from build123d import *

# Parameters (mm, degrees)
BOSS_EXTRUDE3_DEPTH      = 62.5
BOSS_EXTRUDE3_DEPTH_BACK = 62.5
SKETCH4_R                = 1.8
CUT_EXTRUDE1_DEPTH       = 62.5
SKETCH5_R                = 1.8
CUT_EXTRUDE2_DEPTH       = 62.5
SKETCH7_W                = 21.5
SKETCH7_H                = 18
CUT_EXTRUDE5_DEPTH       = 62.5
SKETCH10_W               = 21.5
SKETCH10_H               = 18
CUT_EXTRUDE7_DEPTH       = 62.5
SKETCH13_W               = 21.5
SKETCH13_H               = 28.5
CUT_EXTRUDE9_DEPTH       = 62.5
SKETCH18_W               = 21.5
SKETCH18_H               = 28.5
CUT_EXTRUDE10_DEPTH      = 62.5
SKETCH20_R               = 1.7
CUT_EXTRUDE11_DEPTH      = 62.5
SKETCH21_R               = 1.7
CUT_EXTRUDE12_DEPTH      = 62.5


with BuildPart() as part:
    # Sketch1 → Boss-Extrude3 (new, two sides: drawn at the far end of the back side and taken through both)
    with BuildSketch(Plane.XY.offset(-BOSS_EXTRUDE3_DEPTH_BACK)):
        Polygon((0, 0), (0, 40), (3.5, 40), (3.5, 3.5), (25, 3.5), (25, 0), align=None)
    extrude(amount=BOSS_EXTRUDE3_DEPTH + BOSS_EXTRUDE3_DEPTH_BACK)

    # Sketch4 → Cut-Extrude1 (cut)
    with BuildSketch(Plane.ZY):
        with Locations((-46.25, 20)):
            Circle(SKETCH4_R)
    extrude(amount=-CUT_EXTRUDE1_DEPTH, mode=Mode.SUBTRACT)

    # Sketch5 → Cut-Extrude2 (cut)
    with BuildSketch(Plane.ZY):
        with Locations((46.25, 20)):
            Circle(SKETCH5_R)
    extrude(amount=-CUT_EXTRUDE2_DEPTH, mode=Mode.SUBTRACT)

    # Sketch7 → Cut-Extrude5 (cut)
    with BuildSketch(Plane(origin=(0, 3.5, 0), x_dir=(1, 0, 0), z_dir=(0, 1, 0))):
        with Locations((14.25, -53.5)):
            Rectangle(SKETCH7_W, SKETCH7_H)
    extrude(amount=-CUT_EXTRUDE5_DEPTH, mode=Mode.SUBTRACT)

    # Sketch10 → Cut-Extrude7 (cut)
    with BuildSketch(Plane(origin=(0, 3.5, 0), x_dir=(1, 0, 0), z_dir=(0, 1, 0))):
        with Locations((14.25, 53.5)):
            Rectangle(SKETCH10_W, SKETCH10_H)
    extrude(amount=-CUT_EXTRUDE7_DEPTH, mode=Mode.SUBTRACT)

    # Sketch13 → Cut-Extrude9 (cut)
    with BuildSketch(Plane(origin=(0, 3.5, 0), x_dir=(1, 0, 0), z_dir=(0, 1, 0))):
        with Locations((14.25, -14.25)):
            Rectangle(SKETCH13_W, SKETCH13_H)
    extrude(amount=-CUT_EXTRUDE9_DEPTH, mode=Mode.SUBTRACT)

    # Sketch18 → Cut-Extrude10 (cut)
    with BuildSketch(Plane(origin=(0, 3.5, 0), x_dir=(1, 0, 0), z_dir=(0, 1, 0))):
        with Locations((14.25, 14.25)):
            Rectangle(SKETCH18_W, SKETCH18_H)
    extrude(amount=-CUT_EXTRUDE10_DEPTH, mode=Mode.SUBTRACT)

    # Sketch20 → Cut-Extrude11 (cut)
    with BuildSketch(Plane(origin=(0, 3.5, 0), x_dir=(1, 0, 0), z_dir=(0, 1, 0))):
        with Locations(Location((17, 36.5, 0), (0, 0, 180))):
            Circle(SKETCH20_R)
    extrude(amount=-CUT_EXTRUDE11_DEPTH, mode=Mode.SUBTRACT)

    # Sketch21 → Cut-Extrude12 (cut)
    with BuildSketch(Plane(origin=(0, 3.5, 0), x_dir=(1, 0, 0), z_dir=(0, 1, 0))):
        with Locations(Location((17, -36.5, 0), (0, 0, 180))):
            Circle(SKETCH21_R)
    extrude(amount=-CUT_EXTRUDE12_DEPTH, mode=Mode.SUBTRACT)


solid = part.part
CAD build for the part. Positions are in the model's coordinates, mm. A direction names the side the tool comes from. Give positions to 0.01 mm unless a question says otherwise; leave off trailing zeros. Order: outer loops, then holes, each group sorted by start corner. A loop starts at its lowest first (then second) coordinate and runs counter-clockwise, first axis right, second up. Notation, with made-up numbers: (65, -14) - (104, -14) arc R22 cw to (104, -5) - close; hole circle Ø2 at (59.5, -32.5). An arc over 180 degrees is marked (long way). Answer in a Markdown table with one row per item.
1. Saw through at A-A, the plane x = 17. Give the cut face in (y, z).
Data:
| item | result |
|---|---|
| outline | (0, -44.5) - (3.5, -44.5) - (3.5, -38.2) - (0, -38.2) - close; (0, -34.8) - (3.5, -34.8) - (3.5, -28.5) - (0, -28.5) - close; (0, 28.5) - (3.5, 28.5) - (3.5, 34.8) - (0, 34.8) - close; (0, 38.2) - (3.5, 38.2) - (3.5, 44.5) - (0, 44.5) - close |
2. Probe probe 1 along Z at (x, y) = (17, 2.15); probe 2 along Z at (x, y) = (22, 3); probe 3 along Y at (x, z) = (1, 46.25). List the from-to ranges inside material, lowest first. Write a range as [from, to].
Data:
| item | result |
|---|---|
| probe 1 | z = [-44.5, -38.2], [-34.8, -28.5], [28.5, 34.8], [38.2, 44.5] |
| probe 2 | z = [-44.5, -28.5], [28.5, 44.5] |
| probe 3 | y = [0, 18.2], [21.8, 40] |
3. Saw through at B-B, the plane z = -46.25. Give the cut face in (x, y), plus the area to 3 significant figures.
Data:
| item | result |
|---|---|
| outline | (0, 0) - (3.5, 0) - (3.5, 18.2) - (0, 18.2) - close; (0, 21.8) - (3.5, 21.8) - (3.5, 40) - (0, 40) - close |
| area | 127 mm² |
4. Tool access for faces 5 (the flat face through (14, 2, -28.5)), 6 (the flat face through (14, 2, -44.5)), 7 (the flat face through (14, 3.5, 36)): list every direction of +Z, -Z, +X, -X, +Y, -Y with a clear straight run to the whole face (end or side of a thin tool).
Data:
| item | result |
|---|---|
| face 5 | +X, +Y, -Y |
| face 6 | -Z, +X, +Y, -Y |
| face 7 | +Z, -Z, +X, +Y |
5. Saw through at C-C, the plane x = 5.75. Give the cut face in (y, z).
Data:
| item | result |
|---|---|
| outline | (0, -44.5) - (3.5, -44.5) - (3.5, -28.5) - (0, -28.5) - close; (0, 28.5) - (3.5, 28.5) - (3.5, 44.5) - (0, 44.5) - close |
6. Saw through at D-D, the plane z = 36.5. Give the cut face in (x, y).
Data:
| item | result |
|---|---|
| outline | (0, 0) - (15.3, 0) - (15.3, 3.5) - (3.5, 3.5) - (3.5, 40) - (0, 40) - close; (18.7, 0) - (25, 0) - (25, 3.5) - (18.7, 3.5) - close |
7. Flat gauge pins, fed straight in: pin 1 (10 mm diameter, centred on x = 20, y = 6, fed in from -Z); pin 2 (3 mm diameter, centred on x = 4.5, z = -49.5, fed in from +Y); pin 3 (1.8 mm diameter, centred on x = 19, y = 2.5, fed in from +Z); pin 4 (6 mm diameter, centred on y = 20, z = 46.25, fed in from +X). Where does each tip first touch, or does it go through?
Data:
| item | result |
|---|---|
| pin 1 | stops at z = -44.5 |
| pin 2 | stops at y = 40 |
| pin 3 | stops at z = 44.5 |
| pin 4 | stops at x = 3.5 |
8. Pull direction Z, two halves, no side cores. Call faces 1 (the cylindrical face through (16.2, 1.8, -38)), 2 (the flat face through (2, 20, -62.5)), 3 (the flat face through (14, 2, 44.5)), 4 (the flat face through (2, 40, -1)): pulls with the +Z half, pulls with the -Z half, needs draft (parallel to the pull), parting line crosses it, or undercut.
Data:
| item | result |
|---|---|
| face 1 | undercut |
| face 2 | pulls with the -Z half |
| face 3 | pulls with the +Z half |
| face 4 | needs draft |
